Input: dimensioned drawing with shaded views. Units: mm. Origin: part minimum x, y, z. A direction names the side the tool comes from. Coordinates: 2 decimals unless noted, no trailing zeros. Order: outer loops, then holes, each group sorted by start corner. A loop starts at its lowest first (then second) coordinate and runs counter-clockwise, first axis right, second up.
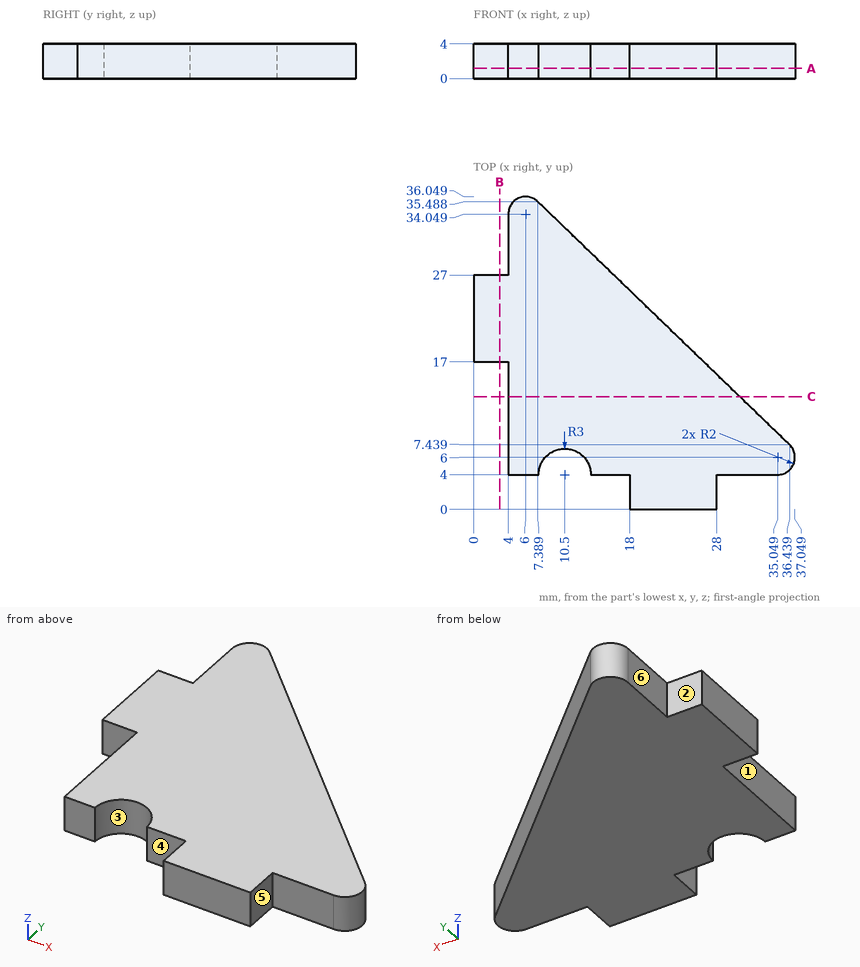
1. Section query C-C, the plane y = 13. Output: boundary loops of the cut face in (x, z), plus the area to 3 significant figures.
2. Material intervals for line 1 along Y through (x, z) = (3, 0.6); line 2 along Y through (x, z) = (5, 0.5); line 3 along X through (y, z) = (13.5, 1.9), sorted ascending.
3. Access query for the marked faces 4, 5 and 6. Directions: +Z, -Z, +X, -X, +Y, -Y. A direction counts if a zero-diameter tool reaches every point of the face in a straight line with its end or side. Return the directions, or none.
4. Contact query for flat-ended pins moving along their axis: P1, Ø1.2, axis at x = 1, z = 3, coming from the +Y side; P2, Ø1.2, axis at x = 3, z = 2.5, coming from the -Y side; P3, Ø2, axis at y = 1, z = 1.5, coming from the +X side. Output: stop coordinate, or through.
5. Section query B-B, the plane x = 3. Output: boundary loops of the cut face in (y, z), plus the area to 3 significant figures.
6. Draft query along X for the marked faces 1, 2 and 3. Return one class per face: +X half, -X half, draft (parallel to the pull), parting line (faces both ways), or undercut.
7. Section query A-A, the plane z = 1.2. Output: boundary loops of the cut face in (x, y).
Answer key:
1. outline: (4, 0) - (30.68, 0) - (30.68, 4) - (4, 4) - close
1. area: 107 mm2
2. line 1: y = 17 to 27
2. line 2: y = 4 to 35.78
2. line 3: x = 4 to 30.16
3. face 4: +Z, -Z, -X, -Y
3. face 5: +Z, -Z, +X, -Y
3. face 6: +Z, -Z, -X, +Y
4. P1: stops at y = 27
4. P2: stops at y = 17
4. P3: stops at x = 28
5. outline: (17, 0) - (27, 0) - (27, 4) - (17, 4) - close
5. area: 40.0 mm2
6. face 1: -X half
6. face 2: draft
6. face 3: undercut
7. outline: (0, 17) - (4, 17) - (4, 4) - (7.5, 4) arc R3 cw to (13.5, 4) - (18, 4) - (18, 0) - (28, 0) - (28, 4) - (35.05, 4) arc R2 ccw to (36.44, 7.44) - (7.39, 35.49) arc R2 ccw to (4, 34.05) - (4, 27) - (0, 27) - close
